Source: three-view drawing plus pictorial views. Frame: mm from the lowest corner of the part. Give positions to 0.01 mm unless a question says otherwise; leave off trailing zeros. Order: outer loops, then holes, each group sorted by start corner. A loop starts at its lowest first (then second) coordinate and runs counter-clockwise, first axis right, second up. Notation, with made-up numbers: (83.25, 49) -> (111.25, 49) arc R4 cw to (111.25, 53) -> close; hole circle Ø10 at (-2.5, 43.25). An arc over 180 degrees is marked (long way). Answer in a Markdown table with one row per item.
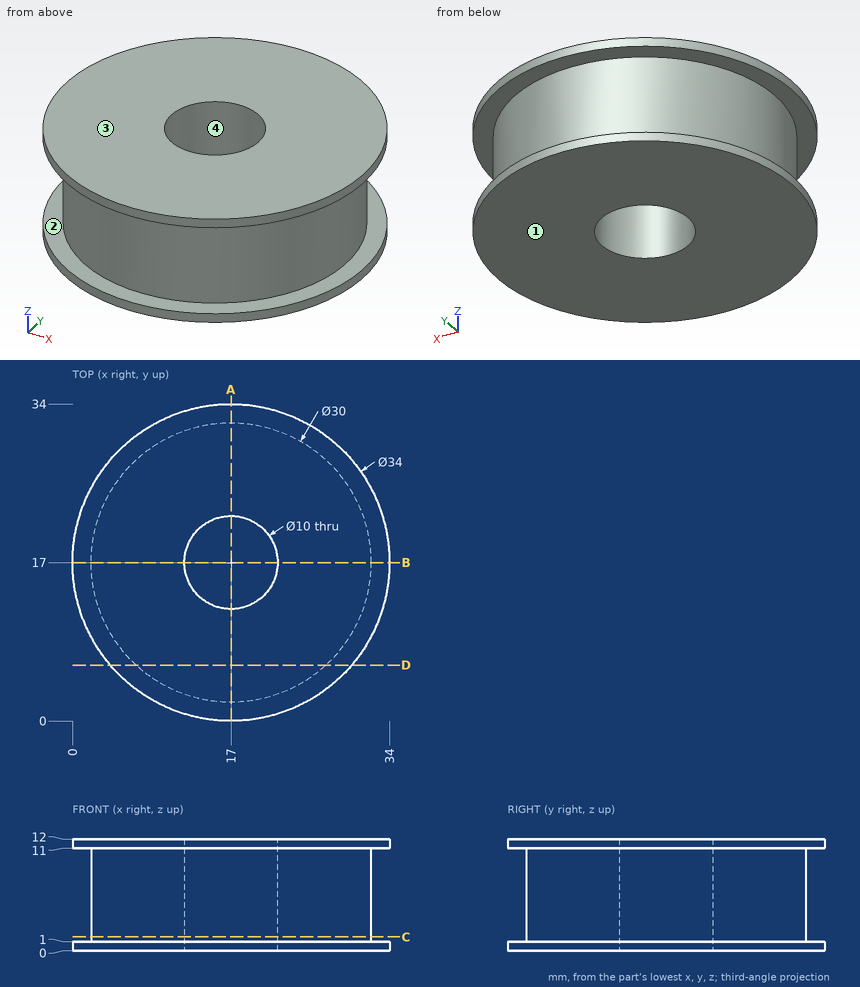
(1) Ray query, probe 1 along Z at (x, y) = (31, 25); probe 2 along Y at (x, z) = (17, 8.5). Return the intervals inside material, ascending.
A:
| item | result |
|---|---|
| probe 1 | z = 0 to 1, 11 to 12 |
| probe 2 | y = 2 to 12, 22 to 32 |
(2) Section query A-A (x = 17). Return the cut outline in (y, z), plus the area to 3 significant figures.
A:
| item | result |
|---|---|
| outline | (0, 0) -> (12, 0) -> (12, 12) -> (0, 12) -> (0, 11) -> (2, 11) -> (2, 1) -> (0, 1) -> close; (22, 0) -> (34, 0) -> (34, 1) -> (32, 1) -> (32, 11) -> (34, 11) -> (34, 12) -> (22, 12) -> close |
| area | 248 mm^2 |
(3) Section query D-D (y = 6). Return the cut outline in (x, z).
A:
| item | result |
|---|---|
| outline | (4.04, 0) -> (29.96, 0) -> (29.96, 1) -> (27.2, 1) -> (27.2, 11) -> (29.96, 11) -> (29.96, 12) -> (4.04, 12) -> (4.04, 11) -> (6.8, 11) -> (6.8, 1) -> (4.04, 1) -> close |
(4) First-contact query: pin 1 Ø2 at (y, z) = (9.5, 5) entering from +X; pin 2 Ø2 at (x, z) = (15, 4.5) entering from -Y; pin 3 Ø1 at (x, z) = (16, 3.5) entering from +Y; pin 4 Ø10 at (x, y) = (18, 20) entering from +Z. Flat tips, straight axial feed; report the tip coordinate or a pass-through.
A:
| item | result |
|---|---|
| pin 1 | stops at x = 30.52 |
| pin 2 | stops at y = 2.03 |
| pin 3 | stops at y = 31.99 |
| pin 4 | stops at z = 12 |
(5) Pull-direction query (Z, two-part tool) for the marked faces 1, 2, 3 and 4; classes: +Z half, -Z half, draft (parallel to the pull), parting line (faces both ways), or undercut.
A:
| item | result |
|---|---|
| face 1 | -Z half |
| face 2 | undercut |
| face 3 | +Z half |
| face 4 | draft |
(6) Section query C-C (z = 1.5). Return the cut outline in (x, y).
A:
| item | result |
|---|---|
| outline | circle Ø30 at (17, 17); hole circle Ø10 at (17, 17) |
